Work out the finished part from the listing and answer in its coordinate system (mm). Face numbers are marked on the shaded views. A direction names the side the tool comes from. Coordinates: 2 decimals unless noted, no trailing zeros. Write each loop counter-clockwise with the first axis right and the second up, starting at its lowest first coordinate (ties: lowest second). Pieces come first, ordered by that corner, then holes. Notation, with made-up numbers: (70, 15.5) - (97, 15.5) arc R19 ccw to (97, 19.5) - close; hole circle Ø3 at (-23.5, 13.25). An arc over 180 degrees is marked (long way). Use one line per item in the form item = value. Start each with the question number.
Item 1: A cutting plane is placed at C-C (z = -8.5). Write down the section's boundary in (x, y).
Item 2: Determine the mould class of the marked faces 3, 4 and 5 for opening direction X: released by +X, released by -X, zero draft, split by the parting line, or undercut.
Item 3: Consider probe 1 along Y at (x, z) = (0, -15.75); probe 2 along Y at (x, z) = (0, 17.5); probe 3 along Z at (x, y) = (-10, -16). Determine where each line is inside the solid, lowest interval first.
Item 4: A cutting plane is placed at B-B (z = 6.5). Write down the section's boundary in (x, y).
Item 5: Given pin 1 (5 mm diameter, centred on y = 10, z = 12.5, fed in from -X); pin 2 (8 mm diameter, centred on x = 0, y = 0, fed in from +Z); pin 3 (2 mm diameter, centred on x = -6.5, z = 0, fed in from -Y), each flat-ended and moving along its own axis, determine where each tip first touches the part or whether it passes through.
Item 6: For the marked faces 1 and 2, determine the directions among +Z, -Z, +X, -X, +Y, -Y from which every point of the face is accessible in a straight line to the end or side of a thin tool.
Item 7: A cutting plane is placed at A-A (z = 14). Write down the section's boundary in (x, y).
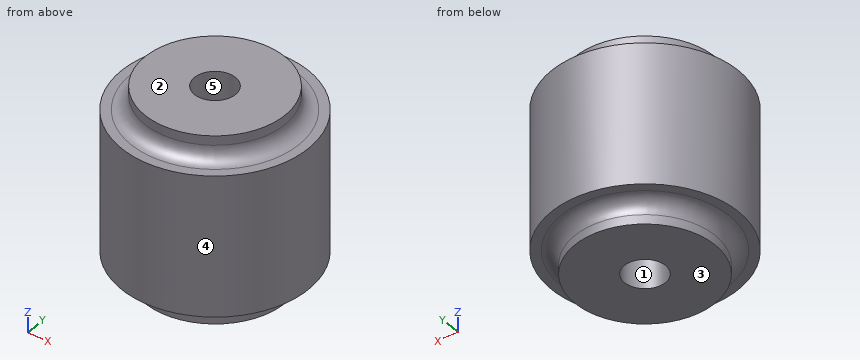
from build123d import *

# Parameters (mm, degrees)
F2_R           = 3
F5_D           = 8.8
F5_DEPTH       = 10
F5_TIP         = 2.6437867237
F5_ON_F3_D     = 8.8
F5_ON_F3_DEPTH = 10
F5_ON_F3_TIP   = 2.6437867237


with BuildPart() as f1:
    # F0 (on Front) → F1 (revolve)
    with BuildSketch(Plane.XZ):
        Polygon((0, -20), (0, 20), (-15, 20), (-15, 15), (-20, 15), (-20, -15), (-15, -15), (-15, -20), align=None)
    revolve(axis=Axis((0, 0, 0), (0, 0, -1)))

    # F2
    f2_edges = [f1.edges().sort_by_distance(p)[0] for p in [
        (15, 0, 15),
        (15, 0, -15),
    ]]
    fillet(f2_edges, radius=F2_R)

    # F5
    with Locations(Plane(origin=(0, 0, -20), x_dir=(1, 0, 0), z_dir=(0, 0, -1))):
        with Locations((0, 0)):
            Hole(F5_D / 2, depth=F5_DEPTH)
            with Locations((0, 0, -(F5_DEPTH + F5_TIP / 2))):  # 118° drill point
                Cone(0, F5_D / 2, F5_TIP, mode=Mode.SUBTRACT)

    # F5 on F3
    with Locations(Plane.XY.offset(20)):
        with Locations((0, 0)):
            Hole(F5_ON_F3_D / 2, depth=F5_ON_F3_DEPTH)
            with Locations((0, 0, -(F5_ON_F3_DEPTH + F5_ON_F3_TIP / 2))):  # 118° drill point
                Cone(0, F5_ON_F3_D / 2, F5_ON_F3_TIP, mode=Mode.SUBTRACT)


solid = f1.part
Answer:
q1.outline = circle Ø40 at (0, 0); hole circle Ø3.81 at (0, 0)
q2.face_3 = zero draft
q2.face_4 = split by the parting line
q2.face_5 = undercut
q3.probe_1 = -16.02 to -4.4, 4.4 to 16.02
q3.probe_2 = -15.04 to -4.4, 4.4 to 15.04
q3.probe_3 = -15 to 15
q4.outline = circle Ø40 at (0, 0)
q5.pin_1 = -18.54
q5.pin_2 = 9.76
q5.pin_3 = -19.23
q6.face_1 = -Z
q6.face_2 = +Z, +X, -X, +Y, -Y
q7.outline = circle Ø40 at (0, 0); hole circle Ø8.8 at (0, 0)
